from build123d import *

# Parameters (mm, degrees)
BOSS_EXTRU_1_DEPTH           = 120
ENL_V_MAT_EXTRU_1_DEPTH      = 243.744721879
ENL_V_MAT_EXTRU_1_DEPTH_BACK = 243.744721879
ENL_V_MAT_EXTRU_2_DEPTH      = 243.744721879
ENL_V_MAT_EXTRU_2_DEPTH_BACK = 243.744721879
ESQUISSE3_R                  = 10
CONG_1_R                     = 20
ENL_V_MAT_EXTRU_3_REACH      = 244.745
ESQUISSE4_R                  = 12.5


with BuildPart() as part:
    # Esquisse1 → Boss.-Extru.1 (new body)
    with BuildSketch(Plane.XY):
        Polygon((0, 0), (0, 205), (50, 205), (50, 0), (45, 0), (45, 200), (5, 200), (5, 0), align=None)
    extrude(amount=BOSS_EXTRU_1_DEPTH)

    # Esquisse2 → Enlèv. mat.-Extru.1 (cut, two sides: drawn at the far end of the back side and taken through both)
    with BuildSketch(Plane(origin=(50, 0, 0), x_dir=(0, 0, -1), z_dir=(1, 0, 0)).offset(-ENL_V_MAT_EXTRU_1_DEPTH_BACK)):
        Polygon((-80, 0), (-120, 125), (-120, 0), align=None)
    extrude(amount=ENL_V_MAT_EXTRU_1_DEPTH + ENL_V_MAT_EXTRU_1_DEPTH_BACK, mode=Mode.SUBTRACT)

    # Esquisse3 → Enlèv. mat.-Extru.2 (cut, two sides: drawn at the far end of the back side and taken through both)
    with BuildSketch(Plane(origin=(50, 0, 0), x_dir=(0, 0, -1), z_dir=(1, 0, 0)).offset(-ENL_V_MAT_EXTRU_2_DEPTH_BACK)):
        with Locations(Location((-40, 30, 0), (0, 0, 90))):
            Circle(ESQUISSE3_R)
    extrude(amount=ENL_V_MAT_EXTRU_2_DEPTH + ENL_V_MAT_EXTRU_2_DEPTH_BACK, mode=Mode.SUBTRACT)

    # Congé1
    cong_1_edges = [part.edges().sort_by_distance(p)[0] for p in [
        (2.5, 125, 120),
        (47.5, 125, 120),
        (2.5, 0, 80),
        (47.5, 0, 80),
        (2.5, 0, 0),
        (47.5, 0, 0),
    ]]
    fillet(cong_1_edges, radius=CONG_1_R)

    # Esquisse4 → Enlèv. mat.-Extru.3 (cut, up to next)
    with BuildSketch(Plane(origin=(0, 205, 0), x_dir=(1, 0, 0), z_dir=(0, 1, 0)), mode=Mode.PRIVATE) as enl_v_mat_extru_3_sk1:
        with Locations(Location((25, -100, 0), (0, 0, 270))):
            Circle(ESQUISSE4_R)
    enl_v_mat_extru_3_tool1 = extrude(enl_v_mat_extru_3_sk1.sketch, amount=-ENL_V_MAT_EXTRU_3_REACH, mode=Mode.PRIVATE) & part.part
    add(enl_v_mat_extru_3_tool1.solids().sort_by_distance((25, 205, 100))[0], mode=Mode.SUBTRACT)


solid = part.part
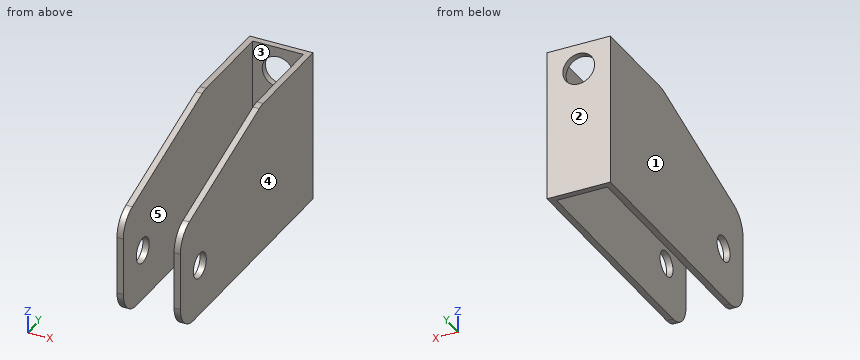
Model file for the job. Use its own axes, mm. Face numbers are marked on the shaded views. A direction names the side the tool comes from. Coordinates: 2 decimals unless noted, no trailing zeros. Write each loop counter-clockwise with the first axis right and the second up, starting at its lowest first coordinate (ties: lowest second). Pieces come first, ordered by that corner, then holes. Notation, with made-up numbers: (-3, 59) - (3, 59) arc R17 ccw to (3, 73) - close; hole circle Ø9 at (-30, 77.5). An arc over 180 degrees is marked (long way). Write each question's results on one line, items separated by ' | '. Start each with the question number.
1) 3-axis set-ups, long thin cutter, end or side, ignore diameter. For the marked faces 4 and 5: which of +Z, -Z, +X, -X, +Y, -Y reach the whole face in a straight line?
2) Cut at B-B (z = 40). Write the cut outline in (x, y).
3) Cut at A-A (y = 119). Write the cut outline in (x, z), then the cut area to 3 significant figures.
4) Cut at C-C (x = 29.5). Write the cut outline in (y, z).
5) Mould opens along X. For the marked faces 1, 2 and 3 say: pulls with the +X half, pulls with the -X half, needs draft (parallel to the pull), parting line crosses it, or undercut.
6) Probe line 1 along X through (y, z) = (16.5, 12.5); line 2 along Y through (x, z) = (3.55, 40); line 3 along X through (y, z) = (202, 100). List the from-to ranges inside material, lowest first. Write a range as from..to.
7) Cut at D-D (z = 100). Write the cut outline in (x, y).
8) Flat gauge pin, fed straight in: P1, Ø8, axis at x = 12, z = 100, coming from the -Y side. Where does the tip first touch, or does it go through?
Returned:
1) face 4: +Z, -Z, +X, +Y, -Y | face 5: +Z, -Z, -Y
2) outline: (0, 0) - (5, 0) - (5, 20) - (0, 20) - close; (0, 40) - (5, 40) - (5, 200) - (45, 200) - (45, 40) - (50, 40) - (50, 205) - (0, 205) - close; (45, 0) - (50, 0) - (50, 20) - (45, 20) - close
3) outline: (0, 0) - (5, 0) - (5, 118.08) - (0, 118.08) - close; (45, 0) - (50, 0) - (50, 118.08) - (45, 118.08) - close | area: 1,180 mm^2
4) outline: (200, 0) - (205, 0) - (205, 88.34) - (200, 88.34) - close; (200, 111.66) - (205, 111.66) - (205, 120) - (200, 120) - close
5) face 1: pulls with the -X half | face 2: needs draft | face 3: undercut
6) line 1: 0..5, 45..50 | line 2: 0..20, 40..205 | line 3: 0..12.5, 37.5..50
7) outline: (0, 62.5) - (5, 62.5) - (5, 200) - (12.5, 200) - (12.5, 205) - (0, 205) - close; (37.5, 200) - (45, 200) - (45, 62.5) - (50, 62.5) - (50, 205) - (37.5, 205) - close
8) P1: y = 200
